Verification items for the finished model (mm, model axes). Coordinates: 2 decimals unless noted, no trailing zeros. Loops run counter-clockwise (first coordinate to the right, second up) from the corner with the lowest first, then second, coordinate; pieces in that order, holes last. Notation, with made-up numbers: (64.5, 70) -> (120.5, 70) arc R21 cw to (120.5, 76) -> close; hole circle Ø10 at (-24, 18.25). An arc over 180 degrees is marked (long way). Write item = value, one per line.
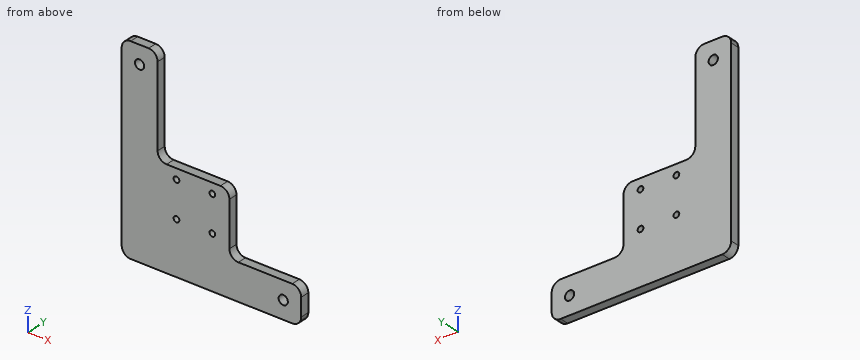
```python
from build123d import *

# Parameters (mm, degrees)
SKETCH1_R                   = 3.2639
BOSS_EXTRUDE1_DEPTH         = 6.35
FILLET1_R                   = 6.35
FILLET4_R                   = 6.35
FILLET5_R                   = 6.35
FILLET6_R                   = 6.35
FILLET9_R                   = 6.35
FILLET10_R                  = 6.35
FILLET11_R                  = 6.35
FILLET12_R                  = 6.35
F_21_0_159_DIAMETER_HOLE1_D = 4.0386


with BuildPart() as part:
    # Sketch1 → Boss-Extrude1 (new body)
    with BuildSketch(Plane(origin=(0, 0, 0), x_dir=(1, 0, 0), z_dir=(0, 1, 0))):
        Polygon((-53.941595929, 54.013787086), (73.058404071, 54.013787086), (73.058404071, 28.613787086), (22.258404071, 28.613787086), (22.258404071, -15.836212914), (-28.541595929, -15.836212914), (-28.541595929, -85.686212914), (-53.941595929, -85.686212914), align=None)
        with Locations((-41.241595929, -72.986212914)):
            Circle(SKETCH1_R, mode=Mode.SUBTRACT)
        with Locations((60.358404071, 41.313787086)):
            Circle(SKETCH1_R, mode=Mode.SUBTRACT)
    extrude(amount=BOSS_EXTRUDE1_DEPTH)

    # Fillet1
    fillet1_edges = [part.edges().sort_by_distance(p)[0] for p in [
        (-28.541595929, 3.175, 15.836212914),
    ]]
    fillet(fillet1_edges, radius=FILLET1_R)

    # Fillet4
    fillet4_edges = [part.edges().sort_by_distance(p)[0] for p in [
        (-53.941595929, 3.175, -54.013787086),
    ]]
    fillet(fillet4_edges, radius=FILLET4_R)

    # Fillet5
    fillet5_edges = [part.edges().sort_by_distance(p)[0] for p in [
        (-53.941595929, 3.175, 85.686212914),
    ]]
    fillet(fillet5_edges, radius=FILLET5_R)

    # Fillet6
    fillet6_edges = [part.edges().sort_by_distance(p)[0] for p in [
        (-28.541595929, 3.175, 85.686212914),
    ]]
    fillet(fillet6_edges, radius=FILLET6_R)

    # Fillet9
    fillet9_edges = [part.edges().sort_by_distance(p)[0] for p in [
        (22.258404071, 3.175, 15.836212914),
    ]]
    fillet(fillet9_edges, radius=FILLET9_R)

    # Fillet10
    fillet10_edges = [part.edges().sort_by_distance(p)[0] for p in [
        (22.258404071, 3.175, -28.613787086),
    ]]
    fillet(fillet10_edges, radius=FILLET10_R)

    # Fillet11
    fillet11_edges = [part.edges().sort_by_distance(p)[0] for p in [
        (73.058404071, 3.175, -28.613787086),
    ]]
    fillet(fillet11_edges, radius=FILLET11_R)

    # Fillet12
    fillet12_edges = [part.edges().sort_by_distance(p)[0] for p in [
        (73.058404071, 3.175, -54.013787086),
    ]]
    fillet(fillet12_edges, radius=FILLET12_R)

    # #21 (0.159) Diameter Hole1 (through all)
    with Locations(Plane(origin=(0, 6.35, 0), x_dir=(1, 0, 0), z_dir=(0, 1, 0))):
        with Locations((-15.182373473, 16.802787086), (-15.182373473, -8.597212914), (10.217626527, -8.597212914), (10.217626527, 16.802787086)):
            Hole(F_21_0_159_DIAMETER_HOLE1_D / 2)


solid = part.part
```
1) Material ranges on line 1 (Z direction, x = 33.5, y = 2.25); line 2 (X direction, y = 1.5, z = 25); line 3 (X direction, y = 2, z = 4), recorded low to high.
Ans:
line_1 = -54.01 to -28.61
line_2 = -53.94 to -28.54
line_3 = -53.94 to 22.26
2) Sectioned sample at A-A, the plane x = 60. Record the cut outline in (y, z), plus the area to 3 significant figures.
Ans:
outline = (0, -54.01) -> (6.35, -54.01) -> (6.35, -44.56) -> (0, -44.56) -> close; (0, -38.07) -> (6.35, -38.07) -> (6.35, -28.61) -> (0, -28.61) -> close
area = 120 mm2
3) Sectioned sample at C-C, the plane z = 28.5. Record the cut outline in (x, y), plus the area to 3 significant figures.
Ans:
outline = (-53.94, 0) -> (-28.54, 0) -> (-28.54, 6.35) -> (-53.94, 6.35) -> close
area = 161 mm2
4) Sectioned sample at D-D, the plane x = -5. Record the cut outline in (y, z), plus the area to 3 significant figures.
Ans:
outline = (0, -54.01) -> (6.35, -54.01) -> (6.35, 15.84) -> (0, 15.84) -> close
area = 444 mm2
5) Depth check by flat-ended pin: pin 1 Ø3 at (y, z) = (2.5, 47) entering from +X; pin 2 Ø2 at (x, y) = (-15, 3.5) entering from +Z; pin 3 Ø1 at (x, y) = (-27.5, 2) entering from +Z. Enter the tip coordinate at first touch or a pass-through.
Ans:
pin_1 = -28.54
pin_2 = 15.84
pin_3 = 19.62
6) Sectioned sample at B-B, the plane y = 4.5. Record the cut outline in (x, z), plus the area to 3 significant figures.
Ans:
outline = (-53.94, -47.66) arc R6.35 ccw to (-47.59, -54.01) -> (66.71, -54.01) arc R6.35 ccw to (73.06, -47.66) -> (73.06, -34.96) arc R6.35 ccw to (66.71, -28.61) -> (28.61, -28.61) arc R6.35 cw to (22.26, -22.26) -> (22.26, 9.49) arc R6.35 ccw to (15.91, 15.84) -> (-22.19, 15.84) arc R6.35 cw to (-28.54, 22.19) -> (-28.54, 79.34) arc R6.35 ccw to (-34.89, 85.69) -> (-47.59, 85.69) arc R6.35 ccw to (-53.94, 79.34) -> close; hole circle Ø6.53 at (-41.24, 72.99); hole circle Ø4.04 at (-15.18, -16.8); hole circle Ø4.04 at (-15.18, 8.6); hole circle Ø4.04 at (10.22, -16.8); hole circle Ø4.04 at (10.22, 8.6); hole circle Ø6.53 at (60.36, -41.31)
area = 8,230 mm2
